Design review of the part built by this model. Coordinates are the model's own, in mm. Round coordinates to 2 decimals unless told otherwise and drop trailing zeros. Loops run counter-clockwise (first coordinate to the right, second up) from the corner with the lowest first, then second, coordinate; pieces in that order, holes last. Notation, with made-up numbers: (89.5, 14.25) - (134.5, 14.25) arc R12 cw to (134.5, 18.25) - close; hole circle Ø3 at (45, 26). An arc over 180 degrees is marked (long way). Return JSON: item names as keys, results as strings. Group by question number.
(1) We need section C-C, the plane x = 9.5. Write out the cut boundary in (y, z), and give its area (3 significant figures).
(2) We need section A-A, the plane z = 0.15. Write out the cut boundary in (x, y).
(3) Wall thickness on L1, parallel to X at y = -0.75, z = 0.1; L2, parallel to X at y = 5.25, z = 0.3; L3, parallel to Y at x = -10, z = 0.9: over which ranges is each line inside the solid? List them lowest first. Write a range as [from, to].
(4) We need section B-B, the plane y = 0. Write out the cut boundary in (x, z), and give its area (3 significant figures).
(5) We need section D-D, the plane x = -9. Write out the cut boundary in (y, z).
(6) The part is to be moulded in two halves that separate along Y. For faces 1 (the cylindrical face through (-7.331, 0.526, 0.507)), 2 (the flat face through (0, -5.77, 0.5)), 3 (the cylindrical face through (-2.953, 5.642, 0.507)), say which applies: pulls with the +Y half, pulls with the -Y half, needs draft (parallel to the pull), parting line crosses it, or undercut.
from build123d import *

# Parameters (mm, degrees)
F4_R     = 1.75
F5_DEPTH = 1


with BuildPart() as f5:
    # F4 (on offset) → F5 (new body, through all)
    with BuildSketch(Plane.XY.offset(1)):
        with BuildLine():
            Line((-4.0505398426, 5.2484339749), (-10.1117136696, 2.2392169874))
            ThreePointArc((-10.1117136696, 2.2392169874), (-11.5, 0), (-10.1117136696, -2.2392169874))
            Line((-10.1117136696, -2.2392169874), (-4.0505398426, -5.2484339749))
            ThreePointArc((-4.0505398426, -5.2484339749), (-2.9690035065, -5.6378624608), (-1.8271125035, -5.77))
            Line((-1.8271125035, -5.77), (0, -5.77))
            Line((0, -5.77), (1.8271125035, -5.77))
            ThreePointArc((1.8271125035, -5.77), (2.9690035065, -5.6378624608), (4.0505398426, -5.2484339749))
            Line((4.0505398426, -5.2484339749), (10.1117136696, -2.2392169874))
            ThreePointArc((10.1117136696, -2.2392169874), (11.5, 0), (10.1117136696, 2.2392169874))
            Line((10.1117136696, 2.2392169874), (4.0505398426, 5.2484339749))
            ThreePointArc((4.0505398426, 5.2484339749), (2.9690035065, 5.6378624608), (1.8271125035, 5.77))
            Line((1.8271125035, 5.77), (0, 5.77))
            Line((0, 5.77), (-1.8271125035, 5.77))
            ThreePointArc((-1.8271125035, 5.77), (-2.9690035065, 5.6378624608), (-4.0505398426, 5.2484339749))
        make_face()
        with Locations((-9, 0)):
            Circle(F4_R, mode=Mode.SUBTRACT)
        with Locations((9, 0)):
            Circle(F4_R, mode=Mode.SUBTRACT)
    extrude(amount=-F5_DEPTH)


solid = f5.part
Solutions:
{
 "1": {"outline": "(-2.54, 0) - (-1.68, 0) - (-1.68, 1) - (-2.54, 1) - close; (1.68, 0) - (2.54, 0) - (2.54, 1) - (1.68, 1) - close", "area": "1.73 mm^2"},
 "2": {"outline": "(-10.11, -2.24) - (-4.05, -5.25) arc R5 ccw to (-1.83, -5.77) - (1.83, -5.77) arc R5 ccw to (4.05, -5.25) - (10.11, -2.24) arc R2.5 ccw to (10.11, 2.24) - (4.05, 5.25) arc R5 ccw to (1.83, 5.77) - (-1.83, 5.77) arc R5 ccw to (-4.05, 5.25) - (-10.11, 2.24) arc R2.5 ccw to start; hole circle Ø3.5 at (-9, 0); hole circle Ø3.5 at (9, 0)"},
 "3": {"L1": "[-11.38, -10.58], [-7.42, 7.42], [10.58, 11.38]", "L2": "[-4.05, 4.05]", "L3": "[-2.29, -1.44], [1.44, 2.29]"},
 "4": {"outline": "(-11.5, 0) - (-10.75, 0) - (-10.75, 1) - (-11.5, 1) - close; (-7.25, 0) - (7.25, 0) - (7.25, 1) - (-7.25, 1) - close; (10.75, 0) - (11.5, 0) - (11.5, 1) - (10.75, 1) - close", "area": "16.0 mm^2"},
 "5": {"outline": "(-2.79, 0) - (-1.75, 0) - (-1.75, 1) - (-2.79, 1) - close; (1.75, 0) - (2.79, 0) - (2.79, 1) - (1.75, 1) - close"},
 "6": {"face 1": "undercut", "face 2": "pulls with the -Y half", "face 3": "pulls with the +Y half"}
}
